Work out the finished part from the listing and answer in its coordinate system (mm). Face numbers are marked on the shaded views. A direction names the side the tool comes from. Coordinates: 2 decimals unless noted, no trailing zeros. Order: outer loops, then holes, each group sorted by start corner. A loop starts at its lowest first (then second) coordinate and runs counter-clockwise, first axis right, second up. Notation, with made-up numbers: M -2.5,18 L 24.5,18 A24 ccw 24.5,53 Z; hole C -16,79.5 d8. An arc over 180 degrees is marked long. Use a Markdown table: item, result. Add a question column.
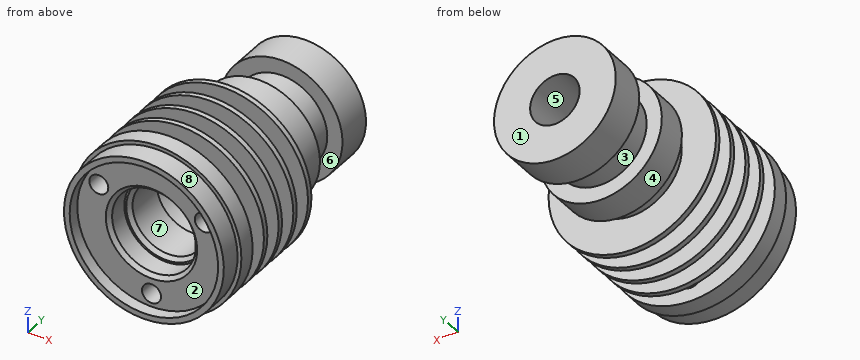
from build123d import *

# Parameters (mm, degrees)
SKETCH2_R                           = 10.5
BOSS_EXTRUDE1_DEPTH                 = 2.8
SKETCH4_W                           = 1.25
SKETCH4_H                           = 5.1
F_2_5_2_5_DIAMETER_HOLE1_AT_2_COUNT = 2
F_2_5_2_5_DIAMETER_HOLE1_AT_2_PITCH = 13.856406461
F_2_5_2_5_DIAMETER_HOLE1_AT_3_COUNT = 2
F_2_5_2_5_DIAMETER_HOLE1_AT_3_PITCH = 13.856406461
CHAMFER1_SIZE                       = 0.5


with BuildPart() as part:
    # Sketch1 → Revolve1 (revolve)
    with BuildSketch(Plane(origin=(0, 0, 0), x_dir=(-1, 0, 0), z_dir=(0, 0, -1)), mode=Mode.PRIVATE) as revolve1_sk:
        Polygon((-11, 2.8), (0, 2.8), (0, 32.9), (-8, 32.9), (-8, 28.1), (-6, 28.1), (-6, 23.5), (-8, 23.5), (-8, 19.4), (-6.5, 19.4), (-6.5, 17.1), (-11, 17.1), (-11, 16.4), (-6.5, 16.4), (-6.5, 14.1), (-11, 14.1), (-11, 13.4), (-6.5, 13.4), (-6.5, 11.1), (-11, 11.1), (-11, 10.4), (-6.5, 10.4), (-6.5, 8.1), (-11, 8.1), (-11, 7.4), (-6.5, 7.4), (-6.5, 5.1), (-11, 5.1), align=None)
    revolve(revolve1_sk.sketch.rotate(Axis((0, 2.8, 0), (0, 1, 0)), 270), axis=Axis((0, 2.8, 0), (0, 1, 0)))

    # Sketch2 → Boss-Extrude1 (add)
    with BuildSketch(Plane.XZ.offset(-2.8)):
        with Locations(Location((0, 0, 0), (0, 0, 270))):
            Circle(SKETCH2_R)
    extrude(amount=BOSS_EXTRUDE1_DEPTH)

    # Sketch3 → Cut-Revolve1 (revolve, cut)
    with BuildSketch(Plane(origin=(0, 0, 0), x_dir=(-1, 0, 0), z_dir=(0, 0, -1)), mode=Mode.PRIVATE) as cut_revolve1_sk:
        Polygon((-9.75, 0), (0, 0), (0, 32.9), (-3.25, 32.9), (-3.25, 11.5), (-4.75, 10), (-4.75, 4.55), (-5.5, 4.55), (-5.5, 1.55), (-9.75, 1.55), align=None)
    revolve(cut_revolve1_sk.sketch.rotate(Axis((0, 0, 0), (0, 1, 0)), 180), axis=Axis((0, 0, 0), (0, 1, 0)), mode=Mode.SUBTRACT)

    # Sketch4 → Ø2.5 (2.5) Diameter Hole1 (revolve, cut)
    with BuildSketch(Plane(origin=(-6.92820323, 5.1, 4), x_dir=(0, 0, 1), z_dir=(1, 0, 0))):
        with Locations((0.625, 2.55)):
            Rectangle(SKETCH4_W, SKETCH4_H)
    f_2_5_2_5_diameter_hole1 = revolve(axis=Axis((-6.92820323, 11.45, 4), (0, -1, 0)), mode=Mode.SUBTRACT)

    # Ø2.5 (2.5) Diameter Hole1 at 2: Ø2.5 (2.5) Diameter Hole1 ×2
    with Locations(*[Vector(0.5000000000000001, 0, -0.8660254037844387) * (i * F_2_5_2_5_DIAMETER_HOLE1_AT_2_PITCH) for i in range(1, F_2_5_2_5_DIAMETER_HOLE1_AT_2_COUNT)]):
        add(f_2_5_2_5_diameter_hole1, mode=Mode.SUBTRACT)

    # Ø2.5 (2.5) Diameter Hole1 at 3: Ø2.5 (2.5) Diameter Hole1 ×2
    with Locations(*[(i * F_2_5_2_5_DIAMETER_HOLE1_AT_3_PITCH, 0, 0) for i in range(1, F_2_5_2_5_DIAMETER_HOLE1_AT_3_COUNT)]):
        add(f_2_5_2_5_diameter_hole1, mode=Mode.SUBTRACT)

    # Chamfer1
    chamfer1_edges = [part.edges().sort_by_distance(p)[0] for p in [
        (4.75, 4.55, 0),
        (5.5, 1.55, 0),
    ]]
    chamfer(chamfer1_edges, length=CHAMFER1_SIZE)


solid = part.part
(1) Which of the six approach directions +Z, -Z, +X, -X, +Y, -Y give full straight-line access (tool end or side, diameter ignored) to the marked faces 1, 2, 3, 4 and 5?
(2) Given P1, Ø5, axis at y = 24, z = 2, coming from the -X side; P2, Ø5, axis at x = -4, y = 17.5, coming from the +Z side; P3, Ø10, axis at y = 28.5, z = -8.5, coming from the -X side, each flat-ended and moving along its own axis, determine where each tip first touches the part or whether it passes through.
(3) Straight lines are drawn through the part: line 1 (Y direction, x = -5.75, z = 6.5); line 2 (Y direction, x = 8, z = 7.25); line 3 (X direction, y = 2.55, z = 4). For each, find the intervals that lie inside material, in ascending order.
(4) The mould has two halves that part along X. Classify the marked faces 6, 7 and 8: pulls with the +X half, pulls with the -X half, needs draft (parallel to the pull), parting line crosses it, or undercut.
(5) A cutting plane is placed at A-A on x = 0. Count the separate pieces of the cut face and the enclosed holes in it, plus the area to 3 significant figures.
(6) A cutting plane is placed at B-B on y = 20.5. Write down the section's boundary in (x, z), plus the area to 3 significant figures.
(7) A cutting plane is placed at C-C on y = 3.5. Write down the section's boundary in (x, z), plus the area to 3 significant figures.
From the geometry:
| question | item | result |
|---|---|---|
| 1 | face 1 | +Z, -Z, +X, -X, +Y |
| 1 | face 2 | -Y |
| 1 | face 3 | none |
| 1 | face 4 | +Y |
| 1 | face 5 | +Y, -Y |
| 2 | P1 | stops at x = -8 |
| 2 | P2 | stops at z = 10.89 |
| 2 | P3 | stops at x = -7.19 |
| 3 | line 1 | y = 1.55 to 5.1, 7.4 to 8.1, 10.4 to 11.1, 13.4 to 14.1, 16.4 to 17.1 |
| 3 | line 2 | y = 2.8 to 5.1, 7.4 to 8.1, 10.4 to 11.1, 13.4 to 14.1, 16.4 to 17.1 |
| 3 | line 3 | x = -9.71 to -8.18, -5.68 to -3.77, 3.77 to 5.68, 8.18 to 9.71 |
| 4 | face 6 | needs draft |
| 4 | face 7 | undercut |
| 4 | face 8 | parting line crosses it |
| 5 | separate pieces | 3 |
| 5 | enclosed holes | 0 |
| 5 | area | 243 mm2 |
| 6 | outline | C 0,0 d16; hole C 0,0 d6.5 |
| 6 | area | 168 mm2 |
| 7 | outline | C 0,0 d22; hole C -6.93,4 d2.5; hole C 0,0 d11; hole C 0,-8 d2.5; hole C 6.93,4 d2.5 |
| 7 | area | 270 mm2 |
